Geometry check sheet. Reference: the model listing, model coordinates, mm. A direction names the side the tool comes from. Round coordinates to 2 decimals unless told otherwise and drop trailing zeros. Write each loop counter-clockwise with the first axis right and the second up, starting at its lowest first coordinate (ties: lowest second). Pieces come first, ordered by that corner, then holes.
Item 1: Cross-section at C-C (z = -40). Enter the section's corners in (x, y).
Item 2: Access from +Z, -Z, +X, -X, +Y, -Y to the whole of each face (thin tool, end or side, straight path). Record for faces 4 (the face through (-21.324, 22.675, -4.032)), 5 (the face through (-1, 67.5, 55)), 6 (the face through (-1, 0, -1)).
Item 3: Depth check by flat-ended pin: P1, Ø7.5, axis at x = 16.5, z = -0.5, coming from the +Y side; P2, Ø19.5, axis at x = 15, z = 0, coming from the +Y side; P3, Ø1.5, axis at x = 29, z = 16.5, coming from the +Y side. Enter the tip coordinate at first touch or a pass-through.
Item 4: Cross-section at B-B (y = 21). Enter the section's corners in (x, z).
Item 5: Cross-section at D-D (y = 102). Enter the section's corners in (x, z), then the cut area to 3 significant figures.
Item 6: Draft check along X on faces 1 (the face through (70, 54, 1)), 2 (the face through (-21, 35, 6)), 3 (the face through (-1, 42, 60)). Enter one of: pulls with the +X half, pulls with the -X half, needs draft (parallel to the pull), parting line crosses it, or undercut.
Item 7: Scan lines: probe 1 along X at (y, z) = (39.25, 0); probe 2 along Z at (x, y) = (0, 101); probe 3 along X at (y, z) = (16.25, 0). Record each from-to range of solid material in increasing order.
Item 8: Cross-section at A-A (x = -15). Enter the section's corners in (y, z), then the cut area to 4 significant figures.
from build123d import *

# Parameters (mm, degrees)
BOX_TOP_VIEW_W                 = 140
BOX_TOP_VIEW_H                 = 120
BOX_EXTRUDE_PART_DEPTH         = 110
INNER_BOX_CUT_W                = 120
INNER_BOX_CUT_H                = 100
INNER_BOX_CUT_1_DEPTH          = 65
SCISSOR_CROSSSECTION_W         = 115
SCISSOR_CROSSSECTION_H         = 15
SCISSOR_CORSSSECTION_CUT_DEPTH = 10
SHAFT_LOCATION_R               = 7.5
SHAFT_LOCATION_CUT_DEPTH       = 35
SKETCH2_R                      = 14
CUT_EXTRUDE2_DEPTH             = 10
M6_TAPPED_HOLE3_AT_2_COUNT     = 2
M6_TAPPED_HOLE3_AT_2_PITCH     = 85.14693183


with BuildPart() as part:
    # Box_top_view → Box_extrude_part (new body)
    with BuildSketch(Plane(origin=(0, 0, 0), x_dir=(1, 0, 0), z_dir=(0, 1, 0))):
        Rectangle(BOX_TOP_VIEW_W, BOX_TOP_VIEW_H)
    extrude(amount=BOX_EXTRUDE_PART_DEPTH)

    # Inner_box_cut → Inner_box_cut_1 (cut)
    with BuildSketch(Plane(origin=(0, 110, 0), x_dir=(1, 0, 0), z_dir=(0, 1, 0))):
        Rectangle(INNER_BOX_CUT_W, INNER_BOX_CUT_H)
    extrude(amount=-INNER_BOX_CUT_1_DEPTH, mode=Mode.SUBTRACT)

    # Scissor_crossSection → Scissor_corssSection_cut (cut)
    with BuildSketch(Plane.XY.offset(60)):
        with Locations((0, 60)):
            Rectangle(SCISSOR_CROSSSECTION_W, SCISSOR_CROSSSECTION_H)
    extrude(amount=-SCISSOR_CORSSSECTION_CUT_DEPTH, mode=Mode.SUBTRACT)

    # Shaft_location → Shaft_location_cut (cut)
    with BuildSketch(Plane(origin=(0, 45, 0), x_dir=(1, 0, 0), z_dir=(0, 1, 0))):
        with Locations(Location((15, 0, 0), (0, 0, 270))):
            Circle(SHAFT_LOCATION_R)
        with Locations(Location((-15, 0, 0), (0, 0, 90))):
            Circle(SHAFT_LOCATION_R)
    extrude(amount=-SHAFT_LOCATION_CUT_DEPTH, mode=Mode.SUBTRACT)

    # Sketch2 → Cut-Extrude2 (cut)
    with BuildSketch(Plane(origin=(0, 45, 0), x_dir=(1, 0, 0), z_dir=(0, 1, 0))):
        with Locations(Location((-15, 0, 0), (0, 0, 270))):
            Circle(SKETCH2_R)
        with Locations(Location((15, 0, 0), (0, 0, 90))):
            Circle(SKETCH2_R)
    extrude(amount=-CUT_EXTRUDE2_DEPTH, mode=Mode.SUBTRACT)

    # Sketch7 → M6 Tapped Hole3 (revolve, cut)
    with BuildSketch(Plane(origin=(0, 110, -55), x_dir=(0, 0, 1), z_dir=(1, 0, 0))):
        Polygon((0, 0), (0, 14.502151548), (2.5, 13), (2.5, 0.525), (3.025, 0), align=None)
    m6_tapped_hole3 = revolve(axis=Axis((0, 116.35, -55), (0, -1, 0)), mode=Mode.SUBTRACT)

    # M6 Tapped Hole3 at 2: M6 Tapped Hole3 ×2
    with Locations(*[Vector(-0.7633862853691146, 0, 0.645942241466174) * (i * M6_TAPPED_HOLE3_AT_2_PITCH) for i in range(1, M6_TAPPED_HOLE3_AT_2_COUNT)]):
        add(m6_tapped_hole3, mode=Mode.SUBTRACT)

    # M6_hole_mirror: M6 Tapped Hole3 across plane
    add(m6_tapped_hole3.mirror(Plane(origin=(0, 0, 0), x_dir=(0, 0, 1), z_dir=(1, 0, 0))), mode=Mode.SUBTRACT)

    # M6_hole_mirror copy 1 sketch → M6_hole_mirror copy 1 (revolve, cut)
    with BuildSketch(Plane(origin=(65, 110, 0), x_dir=(0, 0, 1), z_dir=(-1, 0, 0))):
        Polygon((0, 0), (0, -14.502151548), (2.5, -13), (2.5, -0.525), (3.025, 0), align=None)
    revolve(axis=Axis((65, 116.35, 0), (0, 1, 0)), mode=Mode.SUBTRACT)

    # M6_hole_mirror at the second plane: M6 Tapped Hole3 across plane
    add(m6_tapped_hole3.mirror(Plane.XY), mode=Mode.SUBTRACT)

    # M6_hole_mirror at the second plane copy → M6_hole_mirror at the second plane c 2 (revolve, cut)
    with BuildSketch(Plane(origin=(-65, 110, 0), x_dir=(0, 0, -1), z_dir=(1, 0, 0))):
        Polygon((0, 0), (0, -14.502151548), (2.5, -13), (2.5, -0.525), (3.025, 0), align=None)
    revolve(axis=Axis((-65, 116.35, 0), (0, 1, 0)), mode=Mode.SUBTRACT)


solid = part.part
Resolved:
1. outline: (-70, 0) - (70, 0) - (70, 110) - (60, 110) - (60, 45) - (-60, 45) - (-60, 110) - (-70, 110) - close
2. face 4: +Y
2. face 5: +Z
2. face 6: +Z, -Z, +X, -X, -Y
3. P1: stops at y = 10
3. P2: stops at y = 35
3. P3: stops at y = 45
4. outline: (-70, -60) - (70, -60) - (70, 60) - (-70, 60) - close; hole circle Ø15 at (-15, 0); hole circle Ø15 at (15, 0)
5. outline: (-70, -60) - (70, -60) - (70, 60) - (-70, 60) - close; hole circle Ø5 at (-65, 0); hole (-60, -50) - (60, -50) - (60, 50) - (-60, 50) - close; hole circle Ø5 at (0, -55); hole circle Ø5 at (0, 55); hole circle Ø5 at (65, 0)
5. area: 4,720 mm2
6. face 1: pulls with the +X half
6. face 2: undercut
6. face 3: needs draft
7. probe 1: x = -70 to -29, -1 to 1, 29 to 70
7. probe 2: z = -60 to -57.5, -52.5 to -50, 50 to 52.5, 57.5 to 60
7. probe 3: x = -70 to -22.5, -7.5 to 7.5, 22.5 to 70
8. outline: (0, -60) - (110, -60) - (110, -50) - (45, -50) - (45, -14) - (35, -14) - (35, -7.5) - (10, -7.5) - (10, 7.5) - (35, 7.5) - (35, 14) - (45, 14) - (45, 50) - (52.5, 50) - (52.5, 60) - (0, 60) - close; (67.5, 50) - (110, 50) - (110, 60) - (67.5, 60) - close
8. area: 5,895 mm2
